from build123d import *

# Parameters (mm, degrees)
F0_R          = 17.85
F1_DEPTH      = 50
F2_R          = 1
F3_DEPTH      = 4
F3_DEPTH_BACK = 56
F4_R          = 6
F5_DEPTH      = 1
F6_W          = 1
F6_H          = 4
F7_DEPTH      = 7
F8_R          = 0.5


with BuildPart() as f1:
    # F0 (on Top) → F1 (new body)
    with BuildSketch(Plane.XY):
        Circle(F0_R)
    extrude(amount=F1_DEPTH)

    # F2 (on Top) → F3 (join, two sides)
    with BuildSketch(Plane.XY) as f3_sk:
        Circle(F2_R)
    extrude(amount=-F3_DEPTH)
    extrude(f3_sk.sketch, amount=F3_DEPTH_BACK)

    # F4 (on Top) → F5 (join)
    with BuildSketch(Plane.XY):
        Circle(F4_R)
    extrude(amount=-F5_DEPTH)

    # F6 (on Top) → F7 (join)
    with BuildSketch(Plane.XY):
        with Locations((-13.8, 0)):
            Rectangle(F6_W, F6_H)
        with Locations((13.8, 0)):
            Rectangle(F6_W, F6_H)
    extrude(amount=-F7_DEPTH)

    # F8
    f8_edges = [f1.edges().sort_by_distance(p)[0] for p in [
        (13.8, -2, -7),
        (-13.8, -2, -7),
        (-13.8, 2, -7),
        (13.8, 2, -7),
    ]]
    fillet(f8_edges, radius=F8_R)


solid = f1.part
Read the model definition and answer for the solid it produces. Units are mm, in the model's axes. A direction names the side the tool comes from. Round coordinates to 2 decimals unless told otherwise and drop trailing zeros. Loops run counter-clockwise (first coordinate to the right, second up) from the corner with the lowest first, then second, coordinate; pieces in that order, holes last.
Q1. Section A-A on x = 0 is taken. Write down the section's boundary in (y, z).
Q2. Section D-D on y = -11.5 is taken. Write down the section's boundary in (x, z).
Q3. Each of these flat-tipped pins is pushed along its axis until it touches: pin 1 (1.2 mm diameter, centred on y = -0.5, z = -3, fed in from +X); pin 2 (10 mm diameter, centred on x = -9, y = -1.5, fed in from -Z); pin 3 (1.6 mm diameter, centred on x = 0, y = 0, fed in from -Z); pin 4 (8 mm diameter, centred on y = 10.5, z = 8.5, fed in from -X). Where does it stop, or does it pass through?
Q4. Section C-C on z = 14.5 is taken. Write down the section's boundary in (x, y), and give its area (3 significant figures).
Q5. Which of the six approach directions +Z, -Z, +X, -X, +Y, -Y give full straight-line access (tool end or side, diameter ignored) to faces 1 (the face through (0, -1, -2)), 2 (the face through (14.3, 0, -3)), 3 (the face through (-14.3, 0, -3)), 4 (the face through (13.3, 0, -3)), 5 (the face through (-17.833, 0.785, 24.65))?
Q6. Consider probe 1 along Z at (x, y) = (4, 9); probe 2 along Z at (x, y) = (5, -2); probe 3 along Y at (x, z) = (-10.5, 10). Determine where each line is inside the solid, lowest interval first.
Q7. Determine the mould class of faces 6 (the face through (0, -1, 53)), 7 (the face through (0, 0, 56)), 8 (the face through (-5.994, 0.264, -0.493)) for opening direction X: released by +X, released by -X, zero draft, split by the parting line, or undercut.
Q8. Section B-B on y = 0 is taken. Write down the section's boundary in (x, z).
Output:
1. outline: (-17.85, 0) - (-6, 0) - (-6, -1) - (-1, -1) - (-1, -4) - (1, -4) - (1, -1) - (6, -1) - (6, 0) - (17.85, 0) - (17.85, 50) - (1, 50) - (1, 56) - (-1, 56) - (-1, 50) - (-17.85, 50) - close
2. outline: (-13.65, 0) - (13.65, 0) - (13.65, 50) - (-13.65, 50) - close
3. pin 1: stops at x = 14.3
3. pin 2: stops at z = -7
3. pin 3: stops at z = -4
3. pin 4: stops at x = -16.62
4. outline: circle Ø35.7 at (0, 0)
4. area: 1,000 mm2
5. face 1: -Z
5. face 2: -Z, +X, +Y, -Y
5. face 3: -Z, -X, +Y, -Y
5. face 4: -Z, +Y, -Y
5. face 5: +Z, -Z
6. probe 1: z = 0 to 50
6. probe 2: z = -1 to 50
6. probe 3: y = -14.44 to 14.44
7. face 6: split by the parting line
7. face 7: zero draft
7. face 8: undercut
8. outline: (-17.85, 0) - (-14.3, 0) - (-14.3, -7) - (-13.3, -7) - (-13.3, 0) - (-6, 0) - (-6, -1) - (-1, -1) - (-1, -4) - (1, -4) - (1, -1) - (6, -1) - (6, 0) - (13.3, 0) - (13.3, -7) - (14.3, -7) - (14.3, 0) - (17.85, 0) - (17.85, 50) - (1, 50) - (1, 56) - (-1, 56) - (-1, 50) - (-17.85, 50) - close
